Geometry: final body of the model. Coordinates: model frame, mm. A direction names the side the tool comes from. Round coordinates to 2 decimals unless told otherwise and drop trailing zeros. Order: outer loops, then holes, each group sorted by start corner. A loop starts at its lowest first (then second) coordinate and runs counter-clockwise, first axis right, second up. Notation, with made-up numbers: (39, -16.5) -> (48, -16.5) arc R25 cw to (48, 4.5) -> close; hole circle Ø6 at (-39.75, 57.25). An arc over 180 degrees is marked (long way). Put each result on its own line as item: value.
```python
from build123d import *

# Parameters (mm, degrees)
BOSS_EXTRUDE1_DEPTH = 254
SKETCH2_W           = 17.759293508
SKETCH2_H           = 6.35
BOSS_EXTRUDE2_DEPTH = 25.4


with BuildPart() as part:
    # Sketch1 → Boss-Extrude1 (new body)
    with BuildSketch(Plane.XY):
        Polygon((0, 0), (6.35, 0), (6.35, 38.1), (57.15, 38.1), (57.15, 0), (63.5, 0), (63.5, 44.45), (57.15, 44.45), (6.35, 44.45), (0, 44.45), align=None)
    extrude(amount=BOSS_EXTRUDE1_DEPTH)

    # Sketch2 → Boss-Extrude2 (add)
    with BuildSketch(Plane.XY.offset(254)):
        with Locations((31.75, 41.275)):
            Rectangle(SKETCH2_W, SKETCH2_H)
    extrude(amount=BOSS_EXTRUDE2_DEPTH)


solid = part.part
```
1. Set-up query: faces 1 (the face through (6, 27, 254)), 2 (the face through (58, 27, 254)), 3 (the face through (31, 38.1, 138)). Return all of +Z, -Z, +X, -X, +Y, -Y with unobstructed straight access to the full face (end or side cutting, diameter ignored); none if empty.
Ans:
face 1: +Z, -X, +Y, -Y
face 2: +Z, +X, +Y, -Y
face 3: +Z, -Z, -Y
2. Cut plane A-A on y = 13. Return loops of the section in (x, z), and give its area (3 significant figures).
Ans:
outline: (0, 0) -> (6.35, 0) -> (6.35, 254) -> (0, 254) -> close; (57.15, 0) -> (63.5, 0) -> (63.5, 254) -> (57.15, 254) -> close
area: 3,230 mm²
3. Cut plane C-C on x = 33.5. Return loops of the section in (y, z).
Ans:
outline: (38.1, 0) -> (44.45, 0) -> (44.45, 279.4) -> (38.1, 279.4) -> close
4. Cut plane D-D on x = 53. Return loops of the section in (y, z), and give its area (3 significant figures).
Ans:
outline: (38.1, 0) -> (44.45, 0) -> (44.45, 254) -> (38.1, 254) -> close
area: 1,610 mm²
5. Cut plane B-B on z = 75. Return loops of the section in (x, y), and give its area (3 significant figures).
Ans:
outline: (0, 0) -> (6.35, 0) -> (6.35, 38.1) -> (57.15, 38.1) -> (57.15, 0) -> (63.5, 0) -> (63.5, 44.45) -> (0, 44.45) -> close
area: 887 mm²
6. Draft query along X for faces 4 (the face through (57.15, 19, 125)), 5 (the face through (22.87, 41, 267)), 6 (the face through (32, 39, 0)), 7 (the face through (6.35, 19, 125)). Return one class per face: +X half, -X half, draft (parallel to the pull), parting line (faces both ways), or undercut.
Ans:
face 4: undercut
face 5: -X half
face 6: draft
face 7: undercut
7. Material intervals for probe 1 along X at (y, z) = (5, 21); probe 2 along Y at (x, z) = (52.5, 205); probe 3 along Z at (x, y) = (8.5, 41.5), sorted ascending.
Ans:
probe 1: 0 to 6.35, 57.15 to 63.5
probe 2: 38.1 to 44.45
probe 3: 0 to 254
8. Contact query for flat-ended pins moving along their axis: P1, Ø7, axis at x = 57, y = 27.5, coming from the +Z side; P2, Ø19, axis at y = 28, z = 87.5, coming from the -X side; P3, Ø8, axis at x = 34, z = 41.5, coming from the -Y side; P4, Ø7, axis at y = 40.5, z = 264, coming from the +X side. Output: stop coordinate, or through.
Ans:
P1: z = 254
P2: x = 0
P3: y = 38.1
P4: x = 40.63
